Autodesk Inventor part; units mm, degrees
ref_plane "YZ Plane" through (0, 0, 0) normal (1, 0, 0) x (0, 1, 0)
ref_plane "XZ Plane" through (0, 0, 0) normal (0, 1, 0) x (-1, 0, 0)
ref_plane "XY Plane" through (0, 0, 0) normal (0, 0, 1) x (1, 0, 0)
sketch "Sketch1" plane through (0, 0, 0) normal (0, 0, 1) x (1, 0, 0)
  line L0 (0, 0) -> (20, 0)
  line L1 (20, 0) -> (20, -1)
  line L2 (20, -1) -> (0, -1)
  line L3 (0, -1) -> (0, 0)
  line L4 (0, 0) -> (-5.1595, 19.323)
  line L5 (-5.1595, 19.323) -> (-6.1257, 19.0651)
  line L6 (-6.1257, 19.0651) -> (-0.9662, -0.258)
  line L7 (-0.9662, -0.258) -> (0, 0)
  circle A0 centre (-0.384, -0.5) radius 0.6304
  dimension "d0" = 20
  dimension "d1" = 1
  dimension "d2" = 104.95
extrude "Extrusion1" add sketch "Sketch1" along normal blind 70 and the other way blind 40
properties part number "scharnierband" material "Brass, Soft Yellow, Welded"
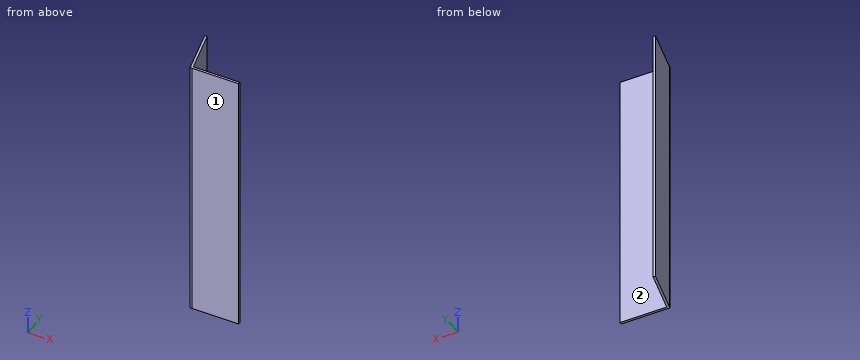
Can you work these out from the model? Positions are in its coordinate system, mm. Face numbers are marked on the shaded views. A direction names the side the tool comes from. Coordinates: 2 decimals unless noted, no trailing zeros. Write each loop counter-clockwise with the first axis right and the second up, starting at its lowest first coordinate (ties: lowest second). Pieces come first, ordered by that corner, then holes. Notation, with made-up numbers: (-5, 18) - (0, 18) arc R8 cw to (0, 33) - close; hole circle Ø6 at (45.25, 84). An arc over 180 degrees is marked (long way). Return JSON: item names as keys, results as strings.
Q1. If we section it at C-C (y = 15.5): Please give me the cut outline in (x, z).
Computed values:
{"outline": "(-5.17, -40) - (-4.14, -40) - (-4.14, 70) - (-5.17, 70) - close"}
Q2. If we section it at B-B (x = 7.75): Please give me the cut outline in (y, z).
Computed values:
{"outline": "(-1, -40) - (0, -40) - (0, 70) - (-1, 70) - close"}
Q3. Please list where these lines run through material, in increasing order: L1, parallel to Y at x = 6.75, z = -23.5; L2, parallel to X at y = 14.5, z = 51; L3, parallel to X at y = 11.5, z = -22. Write a range as from..to.
Computed values:
{"L1": "y = -1..0", "L2": "x = -4.91..-3.87", "L3": "x = -4.11..-3.07"}
Q4. I'm going to push flat-ended pins straight in: pin 1 Ø12 at (x, y) = (3.5, 5) entering from -Z; pin 2 Ø1 at (x, z) = (12, 54) entering from +Y; pin 3 Ø5 at (x, z) = (17, 45) entering from -Y. Where does each tip first touch, or does it pass through?
Computed values:
{"pin 1": "stops at z = -40", "pin 2": "stops at y = 0", "pin 3": "stops at y = -1"}
Q5. If we section it at A-A (z = 59.5): Please give me the cut outline in (x, y), then the cut area to 3 significant figures.
Computed values:
{"outline": "(-6.13, 19.07) - (-0.97, -0.26) arc R0.63 ccw to (0, -1) - (20, -1) - (20, 0) - (0, 0) - (-5.16, 19.32) - close", "area": "40.9 mm2"}
Q6. On a 3-axis mill with a long thin cutter (end or side, diameter ignored), from which of +Z, -Z, +X, -X, +Y, -Y can I reach the whole of each face in a straight line? I mean the marked faces 1 and 2. Say none if no direction works.
Computed values:
{"face 1": "+Z, -Z, +X, -Y", "face 2": "+Z, -Z, +X, +Y"}
